from build123d import *

# Parameters (mm, degrees)
F0_R          = 3.81
F1_DEPTH      = 7.62
F2_R          = 5.08
F3_DEPTH      = 60.96
F4_R          = 3.81
F5_DEPTH      = 7.62
F6_R          = 3.175
F7_DEPTH      = 25.4
F7_DEPTH_BACK = 25.4
F8_R          = 2.54
F9_DEPTH      = 76.201


with BuildPart() as f1:
    # F0 (on Top) → F1 (new body)
    with BuildSketch(Plane.XY):
        Circle(F0_R)
    extrude(amount=F1_DEPTH)

    # F2 (on face) → F3 (join)
    with BuildSketch(Plane.XY.offset(7.62)):
        Circle(F2_R)
    extrude(amount=F3_DEPTH)

    # F4 (on face) → F5 (join)
    with BuildSketch(Plane.XY.offset(68.58)):
        Circle(F4_R)
    extrude(amount=F5_DEPTH)

    # F6 (on Front) → F7 (cut, two sides)
    with BuildSketch(Plane.XZ) as f7_sk:
        with Locations((0, 38.1)):
            Circle(F6_R)
    extrude(amount=-F7_DEPTH, mode=Mode.SUBTRACT)
    extrude(f7_sk.sketch, amount=F7_DEPTH_BACK, mode=Mode.SUBTRACT)

    # F8 (on face) → F9 (cut, through all)
    with BuildSketch(Plane(origin=(0, 0, 0), x_dir=(1, 0, 0), z_dir=(0, 0, -1))):
        Circle(F8_R)
    extrude(amount=-F9_DEPTH, mode=Mode.SUBTRACT)


solid = f1.part
Verification items for the finished model (mm, model axes). A direction names the side the tool comes from. Round coordinates to 2 decimals unless told otherwise and drop trailing zeros. Order: outer loops, then holes, each group sorted by start corner. A loop starts at its lowest first (then second) coordinate and runs counter-clockwise, first axis right, second up.
1. Section check A-A on x = 0. Record the cut outline in (y, z) (3 decimals), then the cut area to 3 significant figures.
Final values:
outline: (-5.08, 7.62) - (-3.81, 7.62) - (-3.81, 0) - (-2.54, 0) - (-2.54, 34.925) - (-5.08, 34.925) - close; (-5.08, 41.275) - (-2.54, 41.275) - (-2.54, 76.2) - (-3.81, 76.2) - (-3.81, 68.58) - (-5.08, 68.58) - close; (2.54, 0) - (3.81, 0) - (3.81, 7.62) - (5.08, 7.62) - (5.08, 34.925) - (2.54, 34.925) - close; (2.54, 41.275) - (5.08, 41.275) - (5.08, 68.58) - (3.81, 68.58) - (3.81, 76.2) - (2.54, 76.2) - close
area: 316 mm2
2. Section check C-C on z = 38.1. Record the cut outline in (x, y) (3 decimals), then the cut area to 3 significant figures.
Final values:
outline: (-3.175, -3.966) - (-3.175, 3.966) arc R5.08 ccw to start; (3.175, -3.966) arc R5.08 ccw to (3.175, 3.966) - close
area: 21.0 mm2
3. Release check for a two-part mould opening along X. For faces 1 (the cylindrical face through (-0.33, -2.52, 57.85)), 2 (the flat face through (0, 3, 0)), 3 (the cylindrical face through (-5.075, 0.223, 37.673)) record: +X half, -X half, draft (parallel to the pull), parting line (faces both ways), or undercut.
Final values:
face 1: undercut
face 2: draft
face 3: parting line
4. Section check B-B on z = 61.5. Record the cut outline in (x, y).
Final values:
outline: circle Ø10.16 at (0, 0); hole circle Ø5.08 at (0, 0)
5. Go/stop test with flat-tipped pins: P1, Ø1, axis at x = 0, y = -2, coming from the -Z side; P2, Ø5, axis at x = -3.5, z = 21, coming from the -Y side. Record where each tip stops, or that it passes through.
Final values:
P1: passes through
P2: stops at y = -4.98
6. Thickness scan on L1, parallel to Y at x = 0.25, z = 17.5; L2, parallel to Z at x = -4.5, y = -1.25; L3, parallel to Y at x = 1.75, z = 20. Record the ranges inside material, lowest first.
Final values:
L1: y = -5.07 to -2.53, 2.53 to 5.07
L2: z = 7.62 to 68.58
L3: y = -4.77 to -1.84, 1.84 to 4.77
7. Access from +Z, -Z, +X, -X, +Y, -Y to the whole of each face (thin tool, end or side, straight path). Record for faces 4 (the cylindrical face through (-0.33, -2.52, 17.84)), 5 (the cylindrical face through (-0.83, -3.72, 72.34)), 6 (the cylindrical face through (-0.83, -3.72, 3.76)).
Final values:
face 4: +Z, -Z
face 5: +Z
face 6: -Z
